For this review, take the finished solid that the model builds, in its own axes (mm). A direction names the side the tool comes from. Give positions to 0.01 mm unless a question says otherwise; leave off trailing zeros. Order: outer loops, then holes, each group sorted by start corner. A loop starts at its lowest first (then second) coordinate and runs counter-clockwise, first axis right, second up.
Item 1: Consider section A-A (y = -19.3). Give the boundary of the cut face in (x, z), plus the area to 3 significant figures.
Item 2: Consider section C-C (z = -7.25). Give the boundary of the cut face in (x, y).
Item 3: Consider section B-B (z = -18). Give the boundary of the cut face in (x, y), plus the area to 3 significant figures.
Item 4: The part is to be moulded in two halves that separate along Z. For faces 3 (the flat face through (0, -13, -20.6)), 4 (the flat face through (0, -27.3, -10)), 5 (the flat face through (0, -5, -5)), say which applies: released by +Z, released by -Z, zero draft, split by the parting line, or undercut.
Item 5: Consider section D-D (y = -8). Give the boundary of the cut face in (x, z).
Item 6: For probe 1 along Z at (x, y) = (-18, -8); probe 2 along Y at (x, z) = (25, -11.25); probe 3 along X at (y, z) = (-18, -1), list the stretches that pass through material, from the lowest coordinate up.
Item 7: Machinability: for faces 1 (the flat face through (0, -13, 0)), 2 (the flat face through (0, -11.3, -10)), which of the approach directions +Z, -Z, +X, -X, +Y, -Y give a long, thin tool a straight path to every point of the face, cutting with its end or side? Answer none if there is none.
```python
from build123d import *

# Parameters (mm, degrees)
SKETCH1_R           = 4
BOSS_EXTRUDE1_DEPTH = 5
BOSS_EXTRUDE2_START = -15.6
SKETCH1_3_R         = 4
BOSS_EXTRUDE2_DEPTH = 10.6
BOSS_EXTRUDE3_START = -15.6
SKETCH1_4_R         = 4
BOSS_EXTRUDE3_DEPTH = 5


with BuildPart() as part:
    # Sketch1 → Boss-Extrude1 (new body)
    # profile 1 of 6: a face of its own
    with BuildSketch(Plane.XY):
        with BuildLine():
            ThreePointArc((-25, -11.3), (-27.58262842, -11.728340311), (-29.888695875, -12.967492389))
            ThreePointArc((-29.888695875, -12.967492389), (-32.571659689, -21.88262842), (-25, -27.3))
            Line((-25, -27.3), (0, -27.3))
            Line((0, -27.3), (0, -11.3))
            Line((0, -11.3), (-25, -11.3))
        make_face()
        with Locations((-25, -19.3)):
            Circle(SKETCH1_R, mode=Mode.SUBTRACT)
    # profile 2 of 6: a face of its own
    with BuildSketch(Plane.XY):
        with BuildLine():
            ThreePointArc((25, -27.3), (32.571659689, -21.88262842), (29.888695875, -12.967492389))
            ThreePointArc((29.888695875, -12.967492389), (27.58262842, -11.728340311), (25, -11.3))
            Line((25, -11.3), (0, -11.3))
            Line((0, -11.3), (0, -27.3))
            Line((0, -27.3), (25, -27.3))
        make_face()
        with Locations((25, -19.3)):
            Circle(SKETCH1_R, mode=Mode.SUBTRACT)
    # profile 3 of 6: a face of its own
    with BuildSketch(Plane.XY):
        with BuildLine():
            Line((29.888695875, -12.967492389), (10.864868878, 1.718902053))
            ThreePointArc((10.864868878, 1.718902053), (10.966165183, 0.862102762), (11, 0))
            ThreePointArc((11, 0), (7.778174593, -7.778174593), (0, -11))
            Line((0, -11), (0, -11.3))
            Line((0, -11.3), (25, -11.3))
            ThreePointArc((25, -11.3), (27.58262842, -11.728340311), (29.888695875, -12.967492389))
        make_face()
    # profile 4 of 6: a face of its own
    with BuildSketch(Plane.XY):
        with BuildLine():
            ThreePointArc((4.888695875, 6.332507611), (2.58262842, 7.571659689), (0, 8))
            Line((0, 8), (0, 3.5))
            ThreePointArc((0, 3.5), (2.474873734, 2.474873734), (3.5, 0))
            ThreePointArc((3.5, 0), (2.474873734, -2.474873734), (0, -3.5))
            Line((0, -3.5), (0, -11))
            ThreePointArc((0, -11), (7.778174593, -7.778174593), (11, 0))
            ThreePointArc((11, 0), (10.966165183, 0.862102762), (10.864868878, 1.718902053))
            Line((10.864868878, 1.718902053), (4.888695875, 6.332507611))
        make_face()
    # profile 5 of 6: a face of its own
    with BuildSketch(Plane.XY):
        with BuildLine():
            Line((0, 3.5), (0, 8))
            ThreePointArc((0, 8), (-2.58262842, 7.571659689), (-4.888695875, 6.332507611))
            Line((-4.888695875, 6.332507611), (-10.864868878, 1.718902053))
            ThreePointArc((-10.864868878, 1.718902053), (-8.363848474, -7.144651056), (0, -11))
            Line((0, -11), (0, -3.5))
            ThreePointArc((0, -3.5), (-3.5, 0), (0, 3.5))
        make_face()
    # profile 6 of 6: a face of its own
    with BuildSketch(Plane.XY):
        with BuildLine():
            ThreePointArc((0, -11), (-8.363848474, -7.144651056), (-10.864868878, 1.718902053))
            Line((-10.864868878, 1.718902053), (-29.888695875, -12.967492389))
            ThreePointArc((-29.888695875, -12.967492389), (-27.58262842, -11.728340311), (-25, -11.3))
            Line((-25, -11.3), (0, -11.3))
            Line((0, -11.3), (0, -11))
        make_face()
    extrude(amount=-BOSS_EXTRUDE1_DEPTH)

    # Sketch1<3> → Boss-Extrude2 (add)
    with BuildSketch(Plane.XY.offset(BOSS_EXTRUDE2_START)):
        with BuildLine():
            Line((-25, -27.3), (25, -27.3))
            ThreePointArc((25, -27.3), (32.571659689, -21.88262842), (29.888695875, -12.967492389))
            ThreePointArc((29.888695875, -12.967492389), (27.58262842, -11.728340311), (25, -11.3))
            Line((25, -11.3), (-25, -11.3))
            ThreePointArc((-25, -11.3), (-27.58262842, -11.728340311), (-29.888695875, -12.967492389))
            ThreePointArc((-29.888695875, -12.967492389), (-32.571659689, -21.88262842), (-25, -27.3))
        make_face()
        with Locations((-25, -19.3)):
            Circle(SKETCH1_3_R, mode=Mode.SUBTRACT)
        with Locations((25, -19.3)):
            Circle(SKETCH1_3_R, mode=Mode.SUBTRACT)
    extrude(amount=BOSS_EXTRUDE2_DEPTH)

    # Sketch1<4> → Boss-Extrude3 (add)
    # profile 1 of 6: a face of its own
    with BuildSketch(Plane.XY.offset(BOSS_EXTRUDE3_START)):
        with BuildLine():
            ThreePointArc((0, -11), (-8.363848474, -7.144651056), (-10.864868878, 1.718902053))
            Line((-10.864868878, 1.718902053), (-29.888695875, -12.967492389))
            ThreePointArc((-29.888695875, -12.967492389), (-27.58262842, -11.728340311), (-25, -11.3))
            Line((-25, -11.3), (0, -11.3))
            Line((0, -11.3), (0, -11))
        make_face()
    # profile 2 of 6: a face of its own
    with BuildSketch(Plane.XY.offset(BOSS_EXTRUDE3_START)):
        with BuildLine():
            Line((0, 3.5), (0, 8))
            ThreePointArc((0, 8), (-2.58262842, 7.571659689), (-4.888695875, 6.332507611))
            Line((-4.888695875, 6.332507611), (-10.864868878, 1.718902053))
            ThreePointArc((-10.864868878, 1.718902053), (-8.363848474, -7.144651056), (0, -11))
            Line((0, -11), (0, -3.5))
            ThreePointArc((0, -3.5), (-3.5, 0), (0, 3.5))
        make_face()
    # profile 3 of 6: a face of its own
    with BuildSketch(Plane.XY.offset(BOSS_EXTRUDE3_START)):
        with BuildLine():
            ThreePointArc((4.888695875, 6.332507611), (2.58262842, 7.571659689), (0, 8))
            Line((0, 8), (0, 3.5))
            ThreePointArc((0, 3.5), (2.474873734, 2.474873734), (3.5, 0))
            ThreePointArc((3.5, 0), (2.474873734, -2.474873734), (0, -3.5))
            Line((0, -3.5), (0, -11))
            ThreePointArc((0, -11), (7.778174593, -7.778174593), (11, 0))
            ThreePointArc((11, 0), (10.966165183, 0.862102762), (10.864868878, 1.718902053))
            Line((10.864868878, 1.718902053), (4.888695875, 6.332507611))
        make_face()
    # profile 4 of 6: a face of its own
    with BuildSketch(Plane.XY.offset(BOSS_EXTRUDE3_START)):
        with BuildLine():
            Line((29.888695875, -12.967492389), (10.864868878, 1.718902053))
            ThreePointArc((10.864868878, 1.718902053), (10.966165183, 0.862102762), (11, 0))
            ThreePointArc((11, 0), (7.778174593, -7.778174593), (0, -11))
            Line((0, -11), (0, -11.3))
            Line((0, -11.3), (25, -11.3))
            ThreePointArc((25, -11.3), (27.58262842, -11.728340311), (29.888695875, -12.967492389))
        make_face()
    # profile 5 of 6: a face of its own
    with BuildSketch(Plane.XY.offset(BOSS_EXTRUDE3_START)):
        with BuildLine():
            ThreePointArc((25, -27.3), (32.571659689, -21.88262842), (29.888695875, -12.967492389))
            ThreePointArc((29.888695875, -12.967492389), (27.58262842, -11.728340311), (25, -11.3))
            Line((25, -11.3), (0, -11.3))
            Line((0, -11.3), (0, -27.3))
            Line((0, -27.3), (25, -27.3))
        make_face()
        with Locations((25, -19.3)):
            Circle(SKETCH1_4_R, mode=Mode.SUBTRACT)
    # profile 6 of 6: a face of its own
    with BuildSketch(Plane.XY.offset(BOSS_EXTRUDE3_START)):
        with BuildLine():
            ThreePointArc((-25, -11.3), (-27.58262842, -11.728340311), (-29.888695875, -12.967492389))
            ThreePointArc((-29.888695875, -12.967492389), (-32.571659689, -21.88262842), (-25, -27.3))
            Line((-25, -27.3), (0, -27.3))
            Line((0, -27.3), (0, -11.3))
            Line((0, -11.3), (-25, -11.3))
        make_face()
        with Locations((-25, -19.3)):
            Circle(SKETCH1_4_R, mode=Mode.SUBTRACT)
    extrude(amount=-BOSS_EXTRUDE3_DEPTH)


solid = part.part
```
Resolved:
1. outline: (-33, -20.6) - (-29, -20.6) - (-29, 0) - (-33, 0) - close; (-21, -20.6) - (21, -20.6) - (21, 0) - (-21, 0) - close; (29, -20.6) - (33, -20.6) - (33, 0) - (29, 0) - close
1. area: 1,030 mm2
2. outline: (-25, -27.3) - (25, -27.3) arc R8 ccw to (25, -11.3) - (-25, -11.3) arc R8 ccw to start; hole circle Ø8 at (-25, -19.3); hole circle Ø8 at (25, -19.3)
3. outline: (-29.89, -12.97) arc R8 ccw to (-25, -27.3) - (25, -27.3) arc R8 ccw to (29.89, -12.97) - (4.89, 6.33) arc R8 ccw to (-4.89, 6.33) - close; hole circle Ø8 at (-25, -19.3); hole circle Ø7 at (0, 0); hole circle Ø8 at (25, -19.3)
3. area: 1,450 mm2
4. face 3: released by -Z
4. face 4: zero draft
4. face 5: undercut
5. outline: (-23.45, -20.6) - (23.45, -20.6) - (23.45, -15.6) - (-23.45, -15.6) - close; (-23.45, -5) - (23.45, -5) - (23.45, 0) - (-23.45, 0) - close
6. probe 1: z = -20.6 to -15.6, -5 to 0
6. probe 2: y = -27.3 to -23.3, -15.3 to -11.3
6. probe 3: x = -32.89 to -28.78, -21.22 to 21.22, 28.78 to 32.89
7. face 1: +Z, +X, -X, +Y, -Y
7. face 2: +X, -X, +Y
